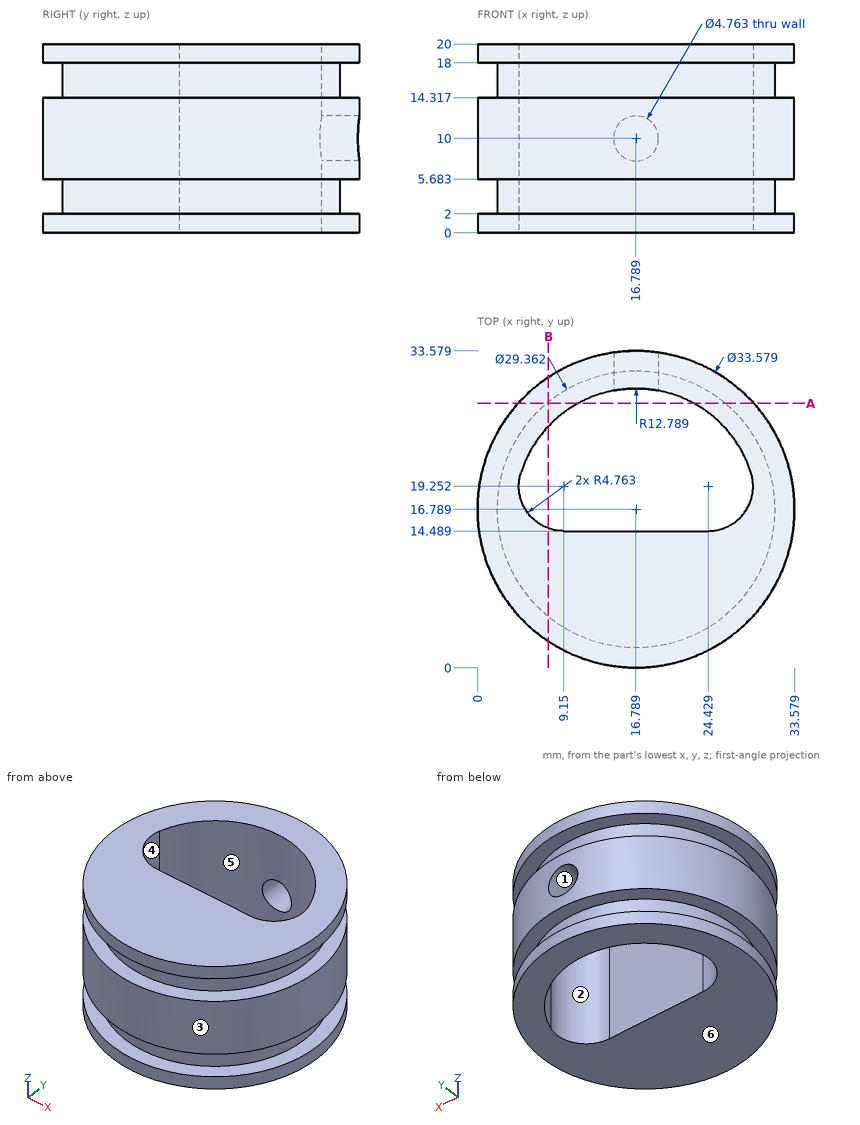
Could you check a few things on this drawing? It's one solid part, dimensions in mm from its lowest x, y, z. A direction names the side the tool comes from. Coordinates: 2 decimals unless noted, no trailing zeros. Order: outer loops, then holes, each group sorted by start corner. A loop starts at its lowest first (then second) coordinate and runs counter-clockwise, first axis right, second up. Notation, with made-up numbers: (-29, 22.25) - (24, 22.25) arc R19 cw to (24, 56.25) - close; hole circle Ø4 at (79.25, -14). An arc over 180 degrees is marked (long way). One line per question, with ' | ' between items. Start each with the question number.
1. If we section it at B-B (x = 7.5): Write out the boundary of the cut face in (y, z) (1 decimal), and give its area (3 significant figures).
2. I'm going to push flat-ended pins straight in: pin 1 Ø12 at (x, z) = (17.5, 12) entering from +Y; pin 2 Ø8 at (y, z) = (12, 15.5) entering from -X; pin 3 Ø5 at (x, z) = (29.5, 2.5) entering from -Y; pin 4 Ø2 at (y, z) = (22, 6) entering from -X. Where does each tip first touch, or does it pass through?
3. If we section it at A-A (y = 28): Write out the boundary of the cut face in (x, z) (1 decimal), and give its area (3 significant figures).
4. Which directions (+Z, -Z, +X, -X, +Y, -Y) give clear straight access to the entire face, cutting with the end or side of a thin tool? Please do the marked faces 5 and 6.
5. Please list where these lines run through material, in increasing order: line 1 along Y through (x, z) = (15, 12.75) (1 decimal); line 2 along Y through (x, z) = (14.5, 4.5); line 3 along X through (y, z) = (18.5, 8). Write a range as [from, to].
6. If we mould it in two halves opening along Y, with no side actions, what happens to the marked faces 1, 2, 3 and 4? For each: released by +Y, released by -Y, zero draft, split by the parting line, or undercut.
Model answer:
1) outline: (2.8, 0) - (14.8, 0) - (14.8, 20) - (2.8, 20) - (2.8, 18) - (5.4, 18) - (5.4, 14.3) - (2.8, 14.3) - (2.8, 5.7) - (5.4, 5.7) - (5.4, 2) - (2.8, 2) - close; (25.6, 0) - (30.8, 0) - (30.8, 2) - (28.2, 2) - (28.2, 5.7) - (30.8, 5.7) - (30.8, 14.3) - (28.2, 14.3) - (28.2, 18) - (30.8, 18) - (30.8, 20) - (25.6, 20) - close | area: 305 mm²
2) pin 1: stops at y = 33.58 | pin 2: stops at x = 0.03 | pin 3: stops at y = 3.5 | pin 4: stops at x = 0.54
3) outline: (4.3, 0) - (10.6, 0) - (10.6, 20) - (4.3, 20) - (4.3, 18) - (7.3, 18) - (7.3, 14.3) - (4.3, 14.3) - (4.3, 5.7) - (7.3, 5.7) - (7.3, 2) - (4.3, 2) - close; (22.9, 0) - (29.3, 0) - (29.3, 2) - (26.3, 2) - (26.3, 5.7) - (29.3, 5.7) - (29.3, 14.3) - (26.3, 14.3) - (26.3, 18) - (29.3, 18) - (29.3, 20) - (22.9, 20) - close | area: 209 mm²
4) face 5: +Z, -Z | face 6: -Z, +X, -X, +Y, -Y
5) line 1: y = [0.1, 14.5], [29.5, 33.5] | line 2: y = [2.29, 14.49], [29.37, 31.29] | line 3: x = [0.09, 4.45], [29.13, 33.49]
6) face 1: zero draft | face 2: undercut | face 3: split by the parting line | face 4: undercut
